from build123d import *

# Parameters (mm, degrees)
BOSS_EXTRUDE1_DEPTH = 24.5
CUT_EXTRUDE1_DEPTH  = 26.12
LPATTERN1_COUNT     = 4
LPATTERN1_PITCH     = 4.5
LPATTERN1_COL_COUNT = 6
LPATTERN1_COL_PITCH = 4.5


with BuildPart() as part:
    # Sketch1 → Boss-Extrude1 (new body)
    with BuildSketch(Plane.XY):
        Polygon((4, 7), (-19, 7), (-19, -0.560353425), (0.939234275, -0.560353425), (40, -0.560353425), (40, 7), align=None)
    extrude(amount=BOSS_EXTRUDE1_DEPTH)

    # Sketch2 → Cut-Extrude1 (cut)
    with BuildSketch(Plane.XY):
        with BuildLine():
            ThreePointArc((-6.881285782, 3.348371163), (-7.417069895, 3.826658598), (-7.671285782, 4.498371163))
            ThreePointArc((-7.671285782, 4.498371163), (-7.912320341, 6.04482582), (-8.981285782, 7.188037328))
            ThreePointArc((-8.981285782, 7.188037328), (-6.881285782, 7.762283268), (-4.781285782, 7.188037328))
            ThreePointArc((-4.781285782, 7.188037328), (-5.850251222, 6.04482582), (-6.091285782, 4.498371163))
            ThreePointArc((-6.091285782, 4.498371163), (-6.345501668, 3.826658598), (-6.881285782, 3.348371163))
        make_face()
    cut_extrude1 = extrude(amount=CUT_EXTRUDE1_DEPTH, mode=Mode.SUBTRACT)

    # LPattern1: Cut-Extrude1 ×4
    with Locations(*[(-i * LPATTERN1_PITCH, 0, 0) for i in range(1, LPATTERN1_COUNT)]):
        add(cut_extrude1, mode=Mode.SUBTRACT)

    # LPattern1 col: Cut-Extrude1 ×6
    with Locations(*[(i * LPATTERN1_COL_PITCH, 0, 0) for i in range(1, LPATTERN1_COL_COUNT)]):
        add(cut_extrude1, mode=Mode.SUBTRACT)


solid = part.part
Geometry check sheet. Reference: the model listing, model coordinates, mm. Give positions to 0.01 mm unless a question says otherwise; leave off trailing zeros. Answer as a JSON object with one key per item and string values.
(1) Draft check along X on faces 1 (the cylindrical face through (11.66, 3.835, 12.078)), 2 (the flat face through (40, 3, 12)), 3 (the flat face through (10, 3, 0)), 4 (the cylindrical face through (15.1, 3.8, 12.1)). Enter one of: released by +X, released by -X, zero draft, split by the parting line, or undercut.
Report:
{"face 1": "undercut", "face 2": "released by +X", "face 3": "zero draft", "face 4": "undercut"}
(2) Cross-section at A-A (y = 5.25). State how many separate pieces and enclosed holes the cut face has, then the cut area to 3 significant figures.
Report:
{"separate pieces": "9", "enclosed holes": "0", "area": "1,140 mm^2"}
(3) Material ranges on line 1 (Y direction, x = 8, z = 4.25); line 2 (Y direction, x = 14.5, z = 23), recorded low to high.
Report:
{"line 1": "-0.56 to 6.59", "line 2": "-0.56 to 6.21"}
